The listing builds one solid part. Answer for the finished solid, in the listing's coordinates (mm). A direction names the side the tool comes from. Round coordinates to 2 decimals unless told otherwise and drop trailing zeros. Write each loop counter-clockwise with the first axis right and the second up, starting at its lowest first coordinate (ties: lowest second). Pieces come first, ordered by that corner, then holes.
from build123d import *

# Parameters (mm, degrees)
SKETCH_13_W         = 27
SKETCH_13_H         = 40
EXTRUDE_11_DEPTH    = 0.5
SKETCH_14_W         = 27
SKETCH_14_H         = 40
EXTRUDE_14_DEPTH    = 1
SKETCH_17_W         = 27
SKETCH_17_H         = 1
EXTRUDE_15_DEPTH    = 0.8
SKETCH_18_R         = 0.8
CUT_EXTRUDE_4_DEPTH = 2
SKETCH_22_W         = 27
SKETCH_22_H         = 1
EXTRUDE_18_DEPTH    = 0.6
SKETCH_23_R         = 0.6
CUT_EXTRUDE_6_DEPTH = 1
SKETCH_24_W         = 1
SKETCH_24_H         = 38
EXTRUDE_19_DEPTH    = 2
SKETCH_25_W         = 1
SKETCH_25_H         = 38
EXTRUDE_20_DEPTH    = 2


with BuildPart() as part:
    # 草图13 → 凸台-拉伸11 (new body)
    with BuildSketch(Plane.XY):
        with Locations((13.5, 20)):
            Rectangle(SKETCH_13_W, SKETCH_13_H)
    extrude(amount=EXTRUDE_11_DEPTH)

    # 草图14 → 凸台-拉伸14 (add)
    with BuildSketch(Plane.XY.offset(0.5)):
        with Locations((13.5, 20)):
            Rectangle(SKETCH_14_W, SKETCH_14_H)
        with BuildLine():
            Line((2, 1), (25, 1))
            ThreePointArc((25, 1), (25.707106781, 1.292893219), (26, 2))
            Line((26, 2), (26, 38))
            ThreePointArc((26, 38), (25.707106781, 38.707106781), (25, 39))
            Line((25, 39), (2, 39))
            ThreePointArc((2, 39), (1.292893219, 38.707106781), (1, 38))
            Line((1, 38), (1, 2))
            ThreePointArc((1, 2), (1.292893219, 1.292893219), (2, 1))
        make_face(mode=Mode.SUBTRACT)
    extrude(amount=EXTRUDE_14_DEPTH)

    # 草图17 → 凸台-拉伸15 (add)
    with BuildSketch(Plane.XY.offset(1.5)):
        with Locations((13.5, 39.5)):
            Rectangle(SKETCH_17_W, SKETCH_17_H)
    extrude(amount=EXTRUDE_15_DEPTH)

    # 草图18 → 切除-拉伸4 (cut, through all)
    with BuildSketch(Plane.XZ.offset(-39)):
        with Locations((13.5, 2.3)):
            Circle(SKETCH_18_R)
    extrude(amount=-CUT_EXTRUDE_4_DEPTH, mode=Mode.SUBTRACT)

    # 草图22 → 凸台-拉伸18 (add)
    with BuildSketch(Plane.XY.offset(1.5)):
        with Locations((13.5, 0.5)):
            Rectangle(SKETCH_22_W, SKETCH_22_H)
    extrude(amount=EXTRUDE_18_DEPTH)

    # 草图23 → 切除-拉伸6 (cut)
    with BuildSketch(Plane.XZ):
        with Locations((13.5, 2.1)):
            Circle(SKETCH_23_R)
    extrude(amount=-CUT_EXTRUDE_6_DEPTH, mode=Mode.SUBTRACT)

    # 草图24 → 凸台-拉伸19 (add)
    with BuildSketch(Plane.XY.offset(1.5)):
        with Locations((26.5, 20)):
            Rectangle(SKETCH_24_W, SKETCH_24_H)
    extrude(amount=EXTRUDE_19_DEPTH)

    # 草图25 → 凸台-拉伸20 (add)
    with BuildSketch(Plane.XY.offset(1.5)):
        with Locations((0.5, 20)):
            Rectangle(SKETCH_25_W, SKETCH_25_H)
    extrude(amount=EXTRUDE_20_DEPTH)


solid = part.part
1. Section B-B on x = 13.5 is taken. Determine the outline of the cut face in (y, z), plus the area to 3 significant figures.
Geometry says:
outline: (0, 0) - (40, 0) - (40, 1.5) - (39, 1.5) - (39, 0.5) - (1, 0.5) - (1, 1.5) - (0, 1.5) - close
area: 22.0 mm2
2. Section A-A on y = 25.5 is taken. Determine the outline of the cut face in (x, z), plus the area to 3 significant figures.
Geometry says:
outline: (0, 0) - (27, 0) - (27, 3.5) - (26, 3.5) - (26, 0.5) - (1, 0.5) - (1, 3.5) - (0, 3.5) - close
area: 19.5 mm2
3. Straight lines are drawn through the part: line 1 along X through (y, z) = (30, 0.8); line 2 along Y through (x, z) = (3.5, 0.75); line 3 along Z through (x, y) = (23.75, 26). For each, find the intervals that lie inside material, in ascending order.
Geometry says:
line 1: x = 0 to 1, 26 to 27
line 2: y = 0 to 1, 39 to 40
line 3: z = 0 to 0.5
4. A tool of negligible diameter and unlimited length cuts with its end or side. For faces 1 (the face through (0.5, 39, 2.9)), 2 (the face through (1, 20, 2)), 3 (the face through (20.5, 0.5, 2.1)), from which of +Z, -Z, +X, -X, +Y, -Y can it reach the whole face along a straight path? Write none if from no direction.
Geometry says:
face 1: +Z, +X, -X, +Y
face 2: +Z
face 3: +Z, +X, -X, -Y
5. For a pull along Y with two mould halves and no side action, classify faces 4 (the face through (1.301, 38.715, 0.993)), 5 (the face through (1.285, 1.301, 0.993)), 6 (the face through (27, 20, 2)), 7 (the face through (13, 40, 1)) as released by +Y, released by -Y, zero draft, split by the parting line, or undercut.
Geometry says:
face 4: undercut
face 5: undercut
face 6: zero draft
face 7: released by +Y
6. Given pin 1 (1.1 mm diameter, centred on x = 5, y = 0.5, fed in from +Z); pin 2 (0.8 mm diameter, centred on x = 0.5, z = 3, fed in from -Y); pin 3 (3 mm diameter, centred on x = 8, y = 7.5, fed in from +Z), each flat-ended and moving along its own axis, determine where each tip first touches the part or whether it passes through.
Geometry says:
pin 1: stops at z = 2.1
pin 2: stops at y = 1
pin 3: stops at z = 0.5
